```python
from build123d import *

# Parameters (mm, degrees)
SKETCH1_R           = 7.5
BOSS_EXTRUDE1_DEPTH = 2
SKETCH2_R           = 6
BOSS_EXTRUDE2_DEPTH = 26
SKETCH3_R           = 5
BOSS_EXTRUDE3_DEPTH = 70
CHAMFER1_SIZE       = 0.2


with BuildPart() as part:
    # Sketch1 → Boss-Extrude1 (new body)
    with BuildSketch(Plane(origin=(0, 0, 0), x_dir=(0, 0, -1), z_dir=(1, 0, 0))):
        Circle(SKETCH1_R)
    extrude(amount=BOSS_EXTRUDE1_DEPTH)

    # Sketch2 → Boss-Extrude2 (add)
    with BuildSketch(Plane(origin=(2, 0, 0), x_dir=(0, 0, -1), z_dir=(1, 0, 0))):
        with Locations(Location((0, 0, 0), (0, 0, 180))):
            Circle(SKETCH2_R)
    extrude(amount=BOSS_EXTRUDE2_DEPTH)

    # Sketch3 → Boss-Extrude3 (add)
    with BuildSketch(Plane(origin=(28, 0, 0), x_dir=(0, 0, -1), z_dir=(1, 0, 0))):
        Circle(SKETCH3_R)
    extrude(amount=BOSS_EXTRUDE3_DEPTH)

    # Chamfer1
    chamfer1_edges = [part.edges().sort_by_distance(p)[0] for p in [
        (0, 0, 7.5),
        (28, 0, -6),
    ]]
    chamfer(chamfer1_edges, length=CHAMFER1_SIZE)


solid = part.part
```
Verification items for the finished model (mm, model axes). A direction names the side the tool comes from. Coordinates: 2 decimals unless noted, no trailing zeros. Write each loop counter-clockwise with the first axis right and the second up, starting at its lowest first coordinate (ties: lowest second). Pieces come first, ordered by that corner, then holes. Notation, with made-up numbers: M -23,67 L -2,67 A30 ccw -2,89 Z; hole C 39.5,-16 d4. An arc over 180 degrees is marked long. Answer as a JSON object with one key per item and string values. Group by question number.
(1) Material ranges on line 1 (X direction, y = -4.5, z = 4.5); line 2 (Y direction, x = 10.5, z = -1.5); line 3 (Z direction, x = 43, y = 3.25), recorded low to high.
(2) Cross-section at A-A, the plane z = 0. Record the cut outline in (x, y).
(3) Tool access check on faces 1 (the face through (28, -5, 2)), 2 (the face through (0, 0, 0)). Record the directions out of +Z, -Z, +X, -X, +Y, -Y that give a thin tool (end or side, any length) a straight path to the whole face; none if there is none.
(4) Cross-section at C-C, the plane x = 72.5. Record the cut outline in (y, z), and give its area (3 significant figures).
(5) Gauge pin test, flat ends, axial feed: pin 1 (8 mm diameter, centred on x = 58, z = -3.5, fed in from -Y); pin 2 (5 mm diameter, centred on x = 67.5, y = -5, fed in from +Z); pin 3 (1.5 mm diameter, centred on x = 10.5, z = 3, fed in from +Y). Record the tip position at first contact, or that the pin passes through.
Reply:
{
 "1": {"line 1": "0 to 2", "line 2": "-5.81 to 5.81", "line 3": "-3.8 to 3.8"},
 "2": {"outline": "M 0,-7.3 L 0.2,-7.5 L 2,-7.5 L 2,-6 L 27.8,-6 L 28,-5.8 L 28,-5 L 98,-5 L 98,5 L 28,5 L 28,5.8 L 27.8,6 L 2,6 L 2,7.5 L 0.2,7.5 L 0,7.3 Z"},
 "3": {"face 1": "+X", "face 2": "+Z, -Z, -X, +Y, -Y"},
 "4": {"outline": "C 0,0 d10", "area": "78.5 mm²"},
 "5": {"pin 1": "y = -5", "pin 2": "z = 4.33", "pin 3": "y = 5.56"}
}
